Build history of the part. All positions in model axes, mm. Round coordinates to 2 decimals unless told otherwise and drop trailing zeros. Loops run counter-clockwise (first coordinate to the right, second up) from the corner with the lowest first, then second, coordinate; pieces in that order, holes last. Notation, with made-up numbers: (26.25, 63.5) -> (85.25, 63.5) arc R19 ccw to (85.25, 69.5) -> close; hole circle Ø1 at (-37, 80). An arc over 180 degrees is marked (long way). Put each result on its own line as item: value. Start each with the question number.
Item 1: Flat gauge pins, fed straight in: pin 1 Ø9 at (x, z) = (-19.05, 9.525) entering from +Y; pin 2 Ø3 at (x, y) = (26.67, 0) entering from +Z. Where does each tip first touch, or does it go through?
Item 2: Cut at D-D, the plane y = -5. List the corners of the cut face in (x, z) (3 decimals), plus the area to 3 significant figures.
Item 3: Cut at B-B, the plane y = 0.75. List the corners of the cut face in (x, z) (3 decimals).
Item 4: Pull direction X, two halves, no side cores. Call faces 1 (the flat face through (-31.75, 0, 9)), 2 (the flat face through (3, 0, 0)), 3 (the cylindrical face through (29.016, -0.973, 9.392)): +X half, -X half, draft (parallel to the pull), parting line (faces both ways), or undercut.
Item 5: Cut at A-A, the plane x = -19.05. List the corners of the cut face in (y, z) (3 decimals), plus the area to 3 significant figures.
Item 6: Cut at C-C, the plane z = 17. List the corners of the cut face in (x, y).
Item 7: Drill centre lines: probe 1 along Z at (x, y) = (-19.05, 0.25) (3 decimals); probe 2 along Y at (x, z) = (26.67, 6); probe 3 along X at (y, z) = (-0.5, 8.25). Where is each one in solid material? Low to high. Write a range as [from, to].
```python
from build123d import *

# Parameters (mm, degrees)
SKETCH1_W           = 63.5
SKETCH1_H           = 12.7
SKETCH1_R           = 2.54
BOSS_EXTRUDE1_DEPTH = 19.05
CUT_EXTRUDE1_REACH  = 14.7
SKETCH2_R           = 3.81
FILLET1_R           = 7.62


with BuildPart() as part:
    # Sketch1 → Boss-Extrude1 (new body)
    with BuildSketch(Plane.XY):
        Rectangle(SKETCH1_W, SKETCH1_H)
        with Locations((26.67, 0)):
            Circle(SKETCH1_R, mode=Mode.SUBTRACT)
    extrude(amount=BOSS_EXTRUDE1_DEPTH)

    # Sketch2 → Cut-Extrude1 (cut, up to next)
    with BuildSketch(Plane(origin=(0, 6.35, 0), x_dir=(1, 0, 0), z_dir=(0, 1, 0)), mode=Mode.PRIVATE) as cut_extrude1_sk1:
        with Locations((-19.05, -9.525)):
            Circle(SKETCH2_R)
    cut_extrude1_tool1 = extrude(cut_extrude1_sk1.sketch, amount=-CUT_EXTRUDE1_REACH, mode=Mode.PRIVATE) & part.part
    add(cut_extrude1_tool1.solids().sort_by_distance((-19.05, 6.35, 9.525))[0], mode=Mode.SUBTRACT)

    # Fillet1
    fillet1_edges = [part.edges().sort_by_distance(p)[0] for p in [
        (-31.75, 0, 19.05),
        (-31.75, 0, 0),
    ]]
    fillet(fillet1_edges, radius=FILLET1_R)


solid = part.part
```
Reply:
1. pin 1: stops at y = 6.35
1. pin 2: passes through
2. outline: (-31.75, 7.62) arc R7.62 ccw to (-24.13, 0) -> (31.75, 0) -> (31.75, 19.05) -> (-24.13, 19.05) arc R7.62 ccw to (-31.75, 11.43) -> close; hole circle Ø7.62 at (-19.05, 9.525)
2. area: 1,140 mm^2
3. outline: (-31.75, 7.62) arc R7.62 ccw to (-24.13, 0) -> (24.243, 0) -> (24.243, 19.05) -> (-24.13, 19.05) arc R7.62 ccw to (-31.75, 11.43) -> close; (29.097, 0) -> (31.75, 0) -> (31.75, 19.05) -> (29.097, 19.05) -> close; hole circle Ø7.62 at (-19.05, 9.525)
4. face 1: -X half
4. face 2: draft
4. face 3: undercut
5. outline: (-6.35, 0) -> (6.35, 0) -> (6.35, 5.715) -> (-6.35, 5.715) -> close; (-6.35, 13.335) -> (6.35, 13.335) -> (6.35, 19.05) -> (-6.35, 19.05) -> close
5. area: 145 mm^2
6. outline: (-29.33, -6.35) -> (31.75, -6.35) -> (31.75, 6.35) -> (-29.33, 6.35) -> close; hole circle Ø5.08 at (26.67, 0)
7. probe 1: z = [0, 5.715], [13.335, 19.05]
7. probe 2: y = [-6.35, -2.54], [2.54, 6.35]
7. probe 3: x = [-31.75, -22.64], [-15.46, 24.18], [29.16, 31.75]
